Input: part model. Units: mm. Frame: model coordinates. A direction names the side the tool comes from. Round coordinates to 2 decimals unless told otherwise and drop trailing zeros. Write each loop counter-clockwise with the first axis right and the second up, starting at its lowest first coordinate (ties: lowest second). Pieces come first, ordered by that corner, then holes. Notation, with made-up numbers: M 17.25,33 L 23.25,33 A21 cw 23.25,44 Z; hole C 59.25,-38 d9. An arc over 180 degrees is marked long. Write each question's results on one line, items separated by ' | '. Start each with the question number.
```python
from build123d import *

# Parameters (mm, degrees)
BOSS_EXTRUDE1_DEPTH = 19.05
SKETCH3_R           = 16.66875
CUT_EXTRUDE1_DEPTH  = 9.525
SKETCH5_R           = 4.9609375
SKETCH5_R_2         = 3.3734375
CUT_EXTRUDE10_DEPTH = 19.05


with BuildPart() as part:
    # Sketch2 → Boss-Extrude1 (new body)
    with BuildSketch(Plane.XY):
        with BuildLine():
            Line((37.846, 0), (927.354, 0))
            ThreePointArc((927.354, 0), (954.115163241, -11.084836759), (965.2, -37.846))
            Line((965.2, -37.846), (965.2, -38.354))
            ThreePointArc((965.2, -38.354), (954.115163241, -65.115163241), (927.354, -76.2))
            Line((927.354, -76.2), (37.846, -76.2))
            ThreePointArc((37.846, -76.2), (11.084836759, -65.115163241), (0, -38.354))
            Line((0, -38.354), (0, -37.846))
            ThreePointArc((0, -37.846), (11.084836759, -11.084836759), (37.846, 0))
        make_face()
    extrude(amount=BOSS_EXTRUDE1_DEPTH)

    # Sketch3 → Cut-Extrude1 (cut)
    with BuildSketch(Plane.XY):
        with Locations((120.65, -38.1)):
            Circle(SKETCH3_R)
        with Locations((241.3, -38.1)):
            Circle(SKETCH3_R)
        with Locations((361.95, -38.1)):
            Circle(SKETCH3_R)
        with Locations((844.55, -38.1)):
            Circle(SKETCH3_R)
        with Locations((723.9, -38.1)):
            Circle(SKETCH3_R)
        with Locations((603.25, -38.1)):
            Circle(SKETCH3_R)
        with Locations((482.6, -38.1)):
            Circle(SKETCH3_R)
    extrude(amount=CUT_EXTRUDE1_DEPTH, mode=Mode.SUBTRACT)

    # Sketch5 → Cut-Extrude10 (cut)
    with BuildSketch(Plane.XY):
        with Locations((38.1, -38.1)):
            Circle(SKETCH5_R)
        with Locations((66.675, -38.1)):
            Circle(SKETCH5_R_2)
        with Locations((62.846675913, -52.3875)):
            Circle(SKETCH5_R_2)
        with Locations((52.3875, -62.846675913)):
            Circle(SKETCH5_R_2)
        with Locations((38.1, -66.675)):
            Circle(SKETCH5_R_2)
        with Locations((23.8125, -62.846675913)):
            Circle(SKETCH5_R_2)
        with Locations((13.353324087, -52.3875)):
            Circle(SKETCH5_R_2)
        with Locations((9.525, -38.1)):
            Circle(SKETCH5_R_2)
        with Locations((13.353324087, -23.8125)):
            Circle(SKETCH5_R_2)
        with Locations((23.8125, -13.353324087)):
            Circle(SKETCH5_R_2)
        with Locations((38.1, -9.525)):
            Circle(SKETCH5_R_2)
        with Locations((52.3875, -13.353324087)):
            Circle(SKETCH5_R_2)
        with Locations((62.846675913, -23.8125)):
            Circle(SKETCH5_R_2)
    extrude(amount=CUT_EXTRUDE10_DEPTH, mode=Mode.SUBTRACT)


solid = part.part
```
1. Cut plane A-A on z = 6. Give the number of separate pieces and of enclosed holes in the cut face, and give its area (3 significant figures).
2. Access query for faces 1 (the face through (954.408, -64.819, 9.392)), 2 (the face through (362, -38, 9.525)). Directions: +Z, -Z, +X, -X, +Y, -Y. A direction counts if a zero-diameter tool reaches every point of the face in a straight line with its end or side. Return the directions, or none.
3. Contact query for flat-ended pins moving along their axis: P1, Ø10, axis at x = 483, y = -42, coming from the -Z side (3 decimals); P2, Ø2, axis at y = -17, z = 5.5, coming from the -X side; P3, Ø16.5, axis at x = 249, y = -44.5, coming from the -Z side; P4, Ø1, axis at y = -46, z = 12, coming from the +X side. Output: stop coordinate, or through.
4. Draft query along X for faces 3 (the face through (489, -38, 19.05)), 4 (the face through (136.55, -33.09, 4.7)), 5 (the face through (10.792, -11.381, 9.392)). Return one class per face: +X half, -X half, draft (parallel to the pull), parting line (faces both ways), or undercut.
5. Line query: L1, parallel to Y at x = 38.1, z = 13.75; L2, parallel to X at y = -65, z = 5.75; L3, parallel to X at y = -12, z = 1. Output: solid intervals per line, ascending. Write a range as from..to.
6. Cut plane B-B on x = 603.25. Output: boundary loops of the cut face in (y, z) (3 decimals), and give its area (3 significant figures).
7. Cut plane C-C on x = 839. Output: boundary loops of the cut face in (y, z) (3 decimals).
Answers follow:
1) separate pieces: 1 | enclosed holes: 20 | area: 65,700 mm2
2) face 1: +Z, -Z, +X, -Y | face 2: -Z
3) P1: stops at z = 9.525 | P2: stops at x = 5.62 | P3: stops at z = 0 | P4: stops at x = 964.52
4) face 3: draft | face 4: undercut | face 5: -X half
5) L1: y = -76.2..-70.05, -63.3..-43.06, -33.14..-12.9, -6.15..0 | L2: x = 10.97..21.22, 26.41..35.17, 41.03..49.79, 54.98..954.23 | L3: x = 10.2..20.72, 26.9..35.81, 40.39..49.3, 55.48..955
6) outline: M -76.2,0 L -54.769,0 L -54.769,9.525 L -21.431,9.525 L -21.431,0 L 0,0 L 0,19.05 L -76.2,19.05 Z | area: 1,130 mm2
7) outline: M -76.2,0 L -53.818,0 L -53.818,9.525 L -22.382,9.525 L -22.382,0 L 0,0 L 0,19.05 L -76.2,19.05 Z
